Model file for the job. Use its own axes, mm. A direction names the side the tool comes from. Give positions to 0.01 mm unless a question says otherwise; leave off trailing zeros. Loops run counter-clockwise (first coordinate to the right, second up) from the corner with the lowest first, then second, coordinate; pieces in that order, holes last. Notation, with made-up numbers: (16, -5) - (30, -5) arc R30 cw to (30, 28) - close; hole circle Ø6 at (-33.5, 23). An arc over 180 degrees is marked (long way). Use a Markdown table: item, result.
from build123d import *

# Parameters (mm, degrees)
BOSS_EXTRU_1_DEPTH = 60
ESQUISSE2_W        = 27
ESQUISSE2_H        = 2063
ESQUISSE2_W_2      = 1046
ESQUISSE2_H_2      = 27
EXTRU_MINCE1_DEPTH = 60


with BuildPart() as part:
    # Esquisse1 → Boss.-Extru.1 (new body)
    with BuildSketch(Plane.XY):
        Polygon((0, 0), (1100, 0), (1100, 1900), (0, 2300), align=None)
        Polygon((27, 27), (1073, 27), (1073, 1881.088463856), (27, 2261.452100219), align=None, mode=Mode.SUBTRACT)
    extrude(amount=BOSS_EXTRU_1_DEPTH)

    # Esquisse2 → Extru.-Mince1 (add)
    with BuildSketch(Plane.XY.offset(60)):
        with Locations((550, 1058.5)):
            Rectangle(ESQUISSE2_W, ESQUISSE2_H)
        with Locations((550, 1881.088463856)):
            Rectangle(ESQUISSE2_W_2, ESQUISSE2_H_2)
        with Locations((550, 981.088463856)):
            Rectangle(ESQUISSE2_W_2, ESQUISSE2_H_2)
    extrude(amount=-EXTRU_MINCE1_DEPTH)


solid = part.part
(1) Slice it at B-B, the plane z = 18.5. Write the cut outline in (x, y) (3 decimals), plus the area to 3 significant figures.
Computed:
| item | result |
|---|---|
| outline | (0, 0) - (1100, 0) - (1100, 1900) - (0, 2300) - close; hole (27, 27) - (536.5, 27) - (536.5, 967.588) - (27, 967.588) - close; hole (27, 994.588) - (536.5, 994.588) - (536.5, 1867.588) - (27, 1867.588) - close; hole (27, 1894.588) - (536.5, 1894.588) - (536.5, 2076.179) - (27, 2261.452) - close; hole (563.5, 27) - (1073, 27) - (1073, 967.588) - (563.5, 967.588) - close; hole (563.5, 994.588) - (1073, 994.588) - (1073, 1867.588) - (563.5, 1867.588) - close; hole (563.5, 1894.588) - (1035.875, 1894.588) - (563.5, 2066.361) - close |
| area | 282,000 mm² |
(2) 3-axis set-ups, long thin cutter, end or side, ignore diameter. For faces 4 (the flat face through (547, 1155, 0)), 5 (the flat face through (278, 967.588, 30)): which of +Z, -Z, +X, -X, +Y, -Y reach the whole face in a straight line?
Computed:
| item | result |
|---|---|
| face 4 | -Z, +X, -X, +Y, -Y |
| face 5 | +Z, -Z |
(3) Mould opens along Y. For faces 1 (the flat face through (0, 1166, 30)), 2 (the flat face through (27, 504, 30)), 3 (the flat face through (542, 0, 30)) say: pulls with the +Y half, pulls with the -Y half, needs draft (parallel to the pull), parting line crosses it, or undercut.
Computed:
| item | result |
|---|---|
| face 1 | needs draft |
| face 2 | undercut |
| face 3 | pulls with the -Y half |
(4) Pin check, flat tip, straight feed: P1, Ø18, axis at x = 230, z = 26, coming from the +Y side. Stop position of the tip, or through.
Computed:
| item | result |
|---|---|
| P1 | y = 2219.64 |
(5) Slice it at D-D, the plane y = 2131. Write the cut outline in (x, z).
Computed:
| item | result |
|---|---|
| outline | (0, 0) - (27, 0) - (27, 60) - (0, 60) - close; (385.74, 0) - (464.75, 0) - (464.75, 60) - (385.74, 60) - close |
(6) Slice it at A-A, the plane y = 229. Write the cut outline in (x, z).
Computed:
| item | result |
|---|---|
| outline | (0, 0) - (27, 0) - (27, 60) - (0, 60) - close; (536.5, 0) - (563.5, 0) - (563.5, 60) - (536.5, 60) - close; (1073, 0) - (1100, 0) - (1100, 60) - (1073, 60) - close |
(7) Slice it at C-C, the plane x = 260.5. Write the cut outline in (y, z).
Computed:
| item | result |
|---|---|
| outline | (0, 0) - (27, 0) - (27, 60) - (0, 60) - close; (967.59, 0) - (994.59, 0) - (994.59, 60) - (967.59, 60) - close; (1867.59, 0) - (1894.59, 0) - (1894.59, 60) - (1867.59, 60) - close; (2176.54, 0) - (2205.27, 0) - (2205.27, 60) - (2176.54, 60) - close |
(8) Drill centre lines: probe 1 along X at (y, z) = (1817.5, 31); probe 2 along Y at (x, z) = (427.5, 11.5); probe 3 along Y at (x, z) = (323, 28.5). Where is each one in solid material? Low to high. Write a range as [from, to].
Computed:
| item | result |
|---|---|
| probe 1 | [0, 27], [536.5, 563.5], [1073, 1100] |
| probe 2 | [0, 27], [967.59, 994.59], [1867.59, 1894.59], [2115.82, 2144.55] |
| probe 3 | [0, 27], [967.59, 994.59], [1867.59, 1894.59], [2153.82, 2182.55] |
